Can you work these out from the model? Positions are in its coordinate system, mm. Face numbers are marked on the shaded views. A direction names the side the tool comes from. Coordinates: 2 decimals unless noted, no trailing zeros. Order: outer loops, then holes, each group sorted by start corner. A loop starts at its lowest first (then second) coordinate and runs counter-clockwise, first axis right, second up. Notation, with made-up numbers: M 12,4.5 L 33,4.5 A24 ccw 33,37.5 Z; hole C 18.5,59 d6. An arc over 180 degrees is marked long. Answer as CSV lines item,"result". Start each with the question number.
1. On a 3-axis mill with a long thin cutter (end or side, diameter ignored), from which of +Z, -Z, +X, -X, +Y, -Y can I reach the whole of each face in a straight line? I mean the marked faces 4, 5, 6, 7 and 8. Say none if no direction works.
2. If we section it at A-A (z = 9.25): List the corners of the cut face in (x, y) for me, plus the area to 3 significant figures.
3. I need wall thicknesses on line 1 along Z through (x, y) = (9.25, -8.25); line 2 along Y through (x, z) = (4.5, 0); line 3 along X through (y, z) = (-9, -0.25). Which ranges of each line are inside material? Lowest first, please. Write a range as from..to.
4. Will these pins go through, and if not, where does the flat tip stop? pin 1 (0.9 mm diameter, centred on y = -9, z = 0, fed in from -X); pin 2 (6.5 mm diameter, centred on y = 0, z = 0, fed in from +X); pin 3 (1.5 mm diameter, centred on x = 10.5, y = 2, fed in from +Z).
5. If we section it at B-B (y = 5.5): List the corners of the cut face in (x, z) for me.
6. If we mould it in two halves opening along Y, with no side actions, what happens to the marked faces 1, 2 and 3? For each: released by +Y, released by -Y, zero draft, split by the parting line, or undercut.
```python
from build123d import *
from build123d.topology import SkipClean

# Parameters (mm, degrees)
BASPROSKE_W         = 12
BASPROSKE_H         = 10.5
TOOTHCUT_DEPTH      = 20.091883092
TEETHCUTS_COUNT     = 19
BORSKE_R            = 2.5
BORE_DEPTH          = 50.0000508
SKETCH1_R           = 5
CUT_EXTRUDE1_DEPTH  = 3
BOSS_EXTRUDE1_DEPTH = 9
SKETCH3_R           = 10.5
SKETCH3_R_2         = 8.249
CUT_EXTRUDE2_DEPTH  = 2


with BuildPart() as part:
    # BasProSke → Base-Revolve (revolve)
    with BuildSketch(Plane(origin=(0, 0, 0), x_dir=(1, 0, 0), z_dir=(0, 1, 0)), mode=Mode.PRIVATE) as base_revolve_sk:
        with Locations((6, 5.25)):
            Rectangle(BASPROSKE_W, BASPROSKE_H)
    revolve(base_revolve_sk.sketch.rotate(Axis((-10, 0, 0), (1, 0, 0)), 180), axis=Axis((-10, 0, 0), (1, 0, 0)))

    # TooCutSke → ToothCut (cut, through all)
    with BuildSketch(Plane(origin=(0, 0, 0), x_dir=(0, 0, -1), z_dir=(1, 0, 0))):
        with BuildLine():
            ThreePointArc((0.505024765, 8.233526036), (0, 8.249), (-0.505024765, 8.233526036))
            ThreePointArc((-0.505024765, 8.233526036), (-0.825185426, 9.406360648), (-1.499357972, 10.41805984))
            ThreePointArc((-1.499357972, 10.41805984), (0, 10.5254), (1.499357972, 10.41805984))
            ThreePointArc((1.499357972, 10.41805984), (0.825185426, 9.406360648), (0.505024765, 8.233526036))
        make_face()
    toothcut = extrude(amount=TOOTHCUT_DEPTH, mode=Mode.SUBTRACT)

    # TeethCuts: ToothCut ×19 about axis
    teethcuts_axis = Axis((0, 0, 0), (1, 0, 0))
    for i in range(1, TEETHCUTS_COUNT):
        add(toothcut.rotate(teethcuts_axis, i * 360 / TEETHCUTS_COUNT), mode=Mode.SUBTRACT)

    # BorSke → Bore (cut, symmetric)
    with BuildSketch(Plane(origin=(0, 0, 0), x_dir=(0, 0, -1), z_dir=(1, 0, 0))):
        with Locations(Location((0, 0, 0), (0, 0, 180))):
            Circle(BORSKE_R)
    extrude(amount=BORE_DEPTH, both=True, mode=Mode.SUBTRACT)

    # Sketch1 → Cut-Extrude1 (cut)
    with BuildSketch(Plane(origin=(12, 0, 0), x_dir=(0, 0, -1), z_dir=(1, 0, 0))):
        Circle(SKETCH1_R)
    extrude(amount=-CUT_EXTRUDE1_DEPTH, mode=Mode.SUBTRACT)

    # Sketch2 → Boss-Extrude1 (add)
    with BuildSketch(Plane(origin=(9, 0, 0), x_dir=(0, 0, -1), z_dir=(1, 0, 0))):
        with BuildLine():
            Line((-2.085372664, -1.378847653), (-2.085372664, 1.378847653))
            ThreePointArc((-2.085372664, 1.378847653), (-2.5, 0), (-2.085372664, -1.378847653))
        make_face()
    extrude(amount=-BOSS_EXTRUDE1_DEPTH)

    # Sketch3 → Cut-Extrude2 (cut)
    with SkipClean():  # the faces are left unmerged after this step: merging them gives an invalid solid
        with BuildSketch(Plane.ZY):
            Circle(SKETCH3_R)
            with Locations(Location((0, 0, 0), (0, 0, 358.773146294))):
                Circle(SKETCH3_R_2, mode=Mode.SUBTRACT)
        extrude(amount=-CUT_EXTRUDE2_DEPTH, mode=Mode.SUBTRACT)


solid = part.part
```
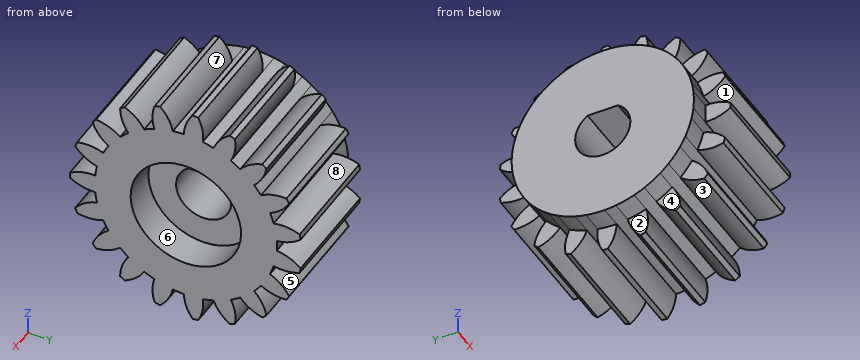
Solved:
1,face 4,"-Z, -X, -Y"
1,face 5,"+X, -X, +Y"
1,face 6,"+X"
1,face 7,"+Z, +X, -X"
1,face 8,"+X, -X"
2,outline,"M 2,-3.01 L 12,-3.01 L 12,-1.57 L 2,-1.57 Z; M 2,-0.02 L 12,-0.02 L 12,1.52 L 2,1.52 Z; M 2,3.41 L 12,3.41 L 12,4.48 L 2,4.48 Z"
2,area,"40.5 mm²"
3,line 1,"-6.5..-5.8, -3.7..-1.92, -0.86..0.86, 1.92..3.7, 5.8..6.5"
3,line 2,"-10.5..-2.5, 2.5..8.25"
3,line 3,"2..12"
4,pin 1,"x = 2"
4,pin 2,"x = 9"
4,pin 3,"z = 10.17"
5,outline,"M 0,-6.15 L 2,-6.15 L 2,-7.18 L 12,-7.18 L 12,7.18 L 2,7.18 L 2,6.15 L 0,6.15 Z"
6,face 1,"released by -Y"
6,face 2,"zero draft"
6,face 3,"undercut"
